Geometry: final body of the model. Coordinates: model frame, mm. A direction names the side the tool comes from. Give positions to 0.01 mm unless a question says otherwise; leave off trailing zeros. Write each loop counter-clockwise with the first axis right and the second up, starting at its lowest first coordinate (ties: lowest second). Pieces come first, ordered by that corner, then holes. Notation, with made-up numbers: M -40,35.5 L 6,35.5 A10 cw 6,54.5 Z; hole C 30.25,31.5 d1. An arc over 180 degrees is marked long. Use a Markdown table: item, result. Add a question column.
1) Section C-C on z = -8.25. Return the cut outline in (x, y).
2) Section B-B on x = -30.5. Return the cut outline in (y, z).
3) Section D-D on x = 13.5. Return the cut outline in (y, z).
4) Pin query (flat end, axial travel): pin 1 (1.8 mm diameter, centred on x = -39, z = -12, fed in from +Y); pin 2 (2 mm diameter, centred on x = -22.5, z = -0.5, fed in from +Y); pin 3 (1.6 mm diameter, centred on x = -21, z = -1, fed in from -Y); pin 4 (3 mm diameter, centred on y = 0, z = -20, fed in from +X). Return the tip coordinate at first contact, or that it passes through.
5) Set-up query: faces 1 (the flat face through (-1, 20.5, -16)), 2 (the flat face through (-6.23, 0, -1)), 3 (the flat face through (40, 0, -16)). Return all of +Z, -Z, +X, -X, +Y, -Y with unobstructed straight access to the full face (end or side cutting, diameter ignored); none if empty.
6) Draft query along Z for faces 4 (the flat face through (-39, 0, -11)), 5 (the flat face through (-1, 23.5, -18)), 6 (the flat face through (-3, -21, -30)). Return one class per face: +Z half, -Z half, draft (parallel to the pull), parting line (faces both ways), or undercut.
7) Line query: line 1 (X direction, y = -12, z = -22.5); line 2 (Y direction, x = 28, z = -6); line 3 (Z direction, x = -8.5, y = 12). Output: solid intervals per line, ascending.
8) Section A-A on z = -20. Return the cut outline in (x, y).
Autodesk Inventor part; units mm, degrees
ref_plane "YZ Plane" through (0, 0, 0) normal (1, 0, 0) x (0, 1, 0)
ref_plane "XZ Plane" through (0, 0, 0) normal (0, 1, 0) x (-1, 0, 0)
ref_plane "XY Plane" through (0, 0, 0) normal (0, 0, 1) x (1, 0, 0)
sketch "Sketch1" plane through (0, 0, 0) normal (0, 0, 1) x (1, 0, 0)
  line L0 (-40, 20.5) -> (40, 20.5)
  line L1 (40, 20.5) -> (40, -20.5)
  line L2 (40, -20.5) -> (-40, -20.5)
  line L3 (-40, -20.5) -> (-40, 20.5)
  line L4 (-40, 20.5) -> (40, -20.5) construction
  line L5 (40, 20.5) -> (-40, -20.5) construction
  line L6 (-43, 23.5) -> (43, 23.5)
  line L7 (43, 23.5) -> (43, -23.5)
  line L8 (43, -23.5) -> (-43, -23.5)
  line L9 (-43, -23.5) -> (-43, 23.5)
  line L10 (-43, 23.5) -> (43, -23.5) construction
  line L11 (43, 23.5) -> (-43, -23.5) construction
  point P0 (0, 0)
  dimension "d0" = 80
  dimension "d1" = 41
  dimension "d2" = 86
  dimension "d3" = 47
extrude "Extrusion1" add sketch "Sketch1" against normal blind 30
sketch "Sketch2" plane through (0, 0, 0) normal (0, 0, 1) x (1, 0, 0)
  line L0 (-40, -20.5) -> (-40, 20.5)
  line L1 (-40, 20.5) -> (40, 20.5)
  line L2 (40, 20.5) -> (40, -20.5)
  line L3 (40, -20.5) -> (-40, -20.5)
  point P0 (0, 0)
extrude "Extrusion2" add sketch "Sketch2" against normal blind 3
sketch "Sketch4" plane through (0, 0, 0) normal (0, 0, 1) x (1, 0, 0)
  line L0 (-43, 23.5) -> (43, 23.5)
  line L1 (-43, -23.5) -> (-43, 23.5)
  line L2 (43, -23.5) -> (-43, -23.5)
  line L3 (43, 23.5) -> (43, -23.5)
  line L4 (-39.5, 20) -> (39.5, 20)
  line L5 (39.5, 20) -> (39.5, -20)
  line L6 (39.5, -20) -> (-39.5, -20)
  line L7 (-39.5, -20) -> (-39.5, 20)
  line L8 (-39.5, 20) -> (39.5, -20) construction
  line L9 (39.5, 20) -> (-39.5, -20) construction
  point P0 (0, 0)
  dimension "d12" = 79
  dimension "d13" = 40
sketch "Sketch5" plane through (0, 0, 0) normal (0, 0, 1) x (1, 0, 0)
  line L0 (-33.23, 9.75) -> (-6.23, 9.75)
  line L1 (-6.23, 9.75) -> (-6.23, -10.25)
  line L2 (-6.23, -10.25) -> (-33.23, -10.25)
  line L3 (-33.23, -10.25) -> (-33.23, 9.75)
  line L4 (-33.23, 9.75) -> (-6.23, -10.25) construction
  line L5 (-6.23, 9.75) -> (-33.23, -10.25) construction
  line L6 (-39.5, 20) -> (39.5, 20)
  line L7 (-39.5, -20) -> (-39.5, 20)
  line L8 (39.5, -20) -> (-39.5, -20)
  point P0 (0, 0)
  point P1 (-19.73, -0.25)
  dimension "d14" = 27
  dimension "d15" = 20
  dimension "d16" = 10.25
  dimension "d17" = 6.27
extrude "Extrusion3" cut sketch "Sketch5" against normal blind 3
sketch "Sketch6" plane through (0, 0, 0) normal (0, 0, 1) x (1, 0, 0)
  circle A0 centre (26.5, 0.5) radius 4
  line L0 (39.5, -20) -> (-39.5, -20)
  line L1 (39.5, 20) -> (39.5, -20)
  line L2 (-39.5, 20) -> (39.5, 20)
  point P0 (0, 0)
  dimension "d20" = 8
  dimension "d21" = 20.5
  dimension "d22" = 13
extrude "Extrusion4" cut sketch "Sketch6" against normal blind 3
chamfer "Chamfer1" distance 1 angle 45 4 edges at (-6.23, -0.25, -3) (-19.73, 9.75, -3) (-19.73, -10.25, -3) (-33.23, -0.25, -3)
chamfer "Chamfer2" distance 1 angle 45 1 edges at (22.5, 0.5, -3)
fillet "Fillet1" radius 6 4 edges at (0, 23.5, 0) (43, 0, 0) (0, -23.5, 0) (-43, 0, 0)
fillet "Fillet2" radius 6 8 edges at (-41.2426, 21.7426, -1.7574) (-43, 23.5, -18) (41.2426, 21.7426, -1.7574) (43, 23.5, -18) (41.2426, -21.7426, -1.7574) (43, -23.5, -18) (-43, -23.5, -18) (-41.2426, -21.7426, -1.7574)
sketch "Sketch7" plane through (-43, -17.5, -6) normal (-1, 0, 0) x (0, 0, 1)
  line L0 (-24, 0) -> (-24, 35)
  circle A0 centre (-14, 17.5) radius 1.75
  point P0 (6, 17.5)
  dimension "d33" = 3.5
  dimension "d34" = 10
extrude "Extrusion5" cut sketch "Sketch7" against normal through all
chamfer "Chamfer3" distance 2 angle 45 2 edges at (-43, 0, -21.75) (43, 0, -21.75)
sketch "Sketch8" plane through (-40, -20.5, -30) normal (1, 0, 0) x (0, 0, -1)
  line L0 (-27, 41) -> (-27, 0)
  line L1 (-19, 36.7314) -> (-16, 36.7314)
  line L2 (-16, 36.7314) -> (-16, 4.7314)
  line L3 (-16, 4.7314) -> (-19, 4.7314)
  line L4 (-19, 4.7314) -> (-19, 36.7314)
  point P0 (-30, 20.5)
  dimension "d40" = 3
  dimension "d41" = 32
  dimension "d42" = 8
extrude "Extrusion6" add sketch "Sketch8" along normal blind 1.6
sketch "Sketch9" plane through (40, -20.5, -30) normal (-1, 0, 0) x (0, 0, 1)
  line L0 (16, 36.7314) -> (19, 36.7314)
  line L1 (19, 36.7314) -> (19, 4.7314)
  line L2 (19, 4.7314) -> (16, 4.7314)
  line L3 (16, 4.7314) -> (16, 36.7314)
  point P0 (30, 20.5)
extrude "Extrusion7" add sketch "Sketch9" along normal blind 1.6
properties part number "obudowa - timer- front"
Found:
| question | item | result |
|---|---|---|
| 1 | outline | M -43,-17.5 A6 ccw -37,-23.5 L 37,-23.5 A6 ccw 43,-17.5 L 43,17.5 A6 ccw 37,23.5 L -37,23.5 A6 ccw -43,17.5 Z; hole M -40,-20.5 L 40,-20.5 L 40,20.5 L -40,20.5 Z |
| 2 | outline | M -23.5,-30 L -20.5,-30 L -20.5,-3 L -11.25,-3 L -10.25,-2 L -10.25,0 L -17.5,0 A6 ccw -23.5,-6 Z; M 9.75,-2 L 10.75,-3 L 20.5,-3 L 20.5,-30 L 23.5,-30 L 23.5,-6 A6 ccw 17.5,0 L 9.75,0 Z |
| 3 | outline | M -23.5,-30 L -20.5,-30 L -20.5,-3 L 20.5,-3 L 20.5,-30 L 23.5,-30 L 23.5,-6 A6 ccw 17.5,0 L -17.5,0 A6 ccw -23.5,-6 Z |
| 4 | pin 1 | y = 23.4 |
| 4 | pin 2 | y = 21.47 |
| 4 | pin 3 | y = -21.78 |
| 4 | pin 4 | through |
| 5 | face 1 | -Z |
| 5 | face 2 | +Z, -Z |
| 5 | face 3 | none |
| 6 | face 4 | undercut |
| 6 | face 5 | draft |
| 6 | face 6 | -Z half |
| 7 | line 1 | -43 to -40, 40 to 43 |
| 7 | line 2 | -23.5 to -20.5, 20.5 to 23.5 |
| 7 | line 3 | -3 to 0 |
| 8 | outline | M -43,-17.5 A6 ccw -37,-23.5 L 37,-23.5 A6 ccw 43,-17.5 L 43,-3.75 L 41,-1.75 L 40,-1.75 L 40,-20.5 L -40,-20.5 L -40,-1.75 L -41,-1.75 L -43,-3.75 Z; M -43,3.75 L -41,1.75 L -40,1.75 L -40,20.5 L 40,20.5 L 40,1.75 L 41,1.75 L 43,3.75 L 43,17.5 A6 ccw 37,23.5 L -37,23.5 A6 ccw -43,17.5 Z |
